Check sheet for the drawn part. Datum: minimum x, y, z corner. Units: mm. A direction names the side the tool comes from. Give positions to 0.01 mm unless a question says otherwise; leave off trailing zeros.
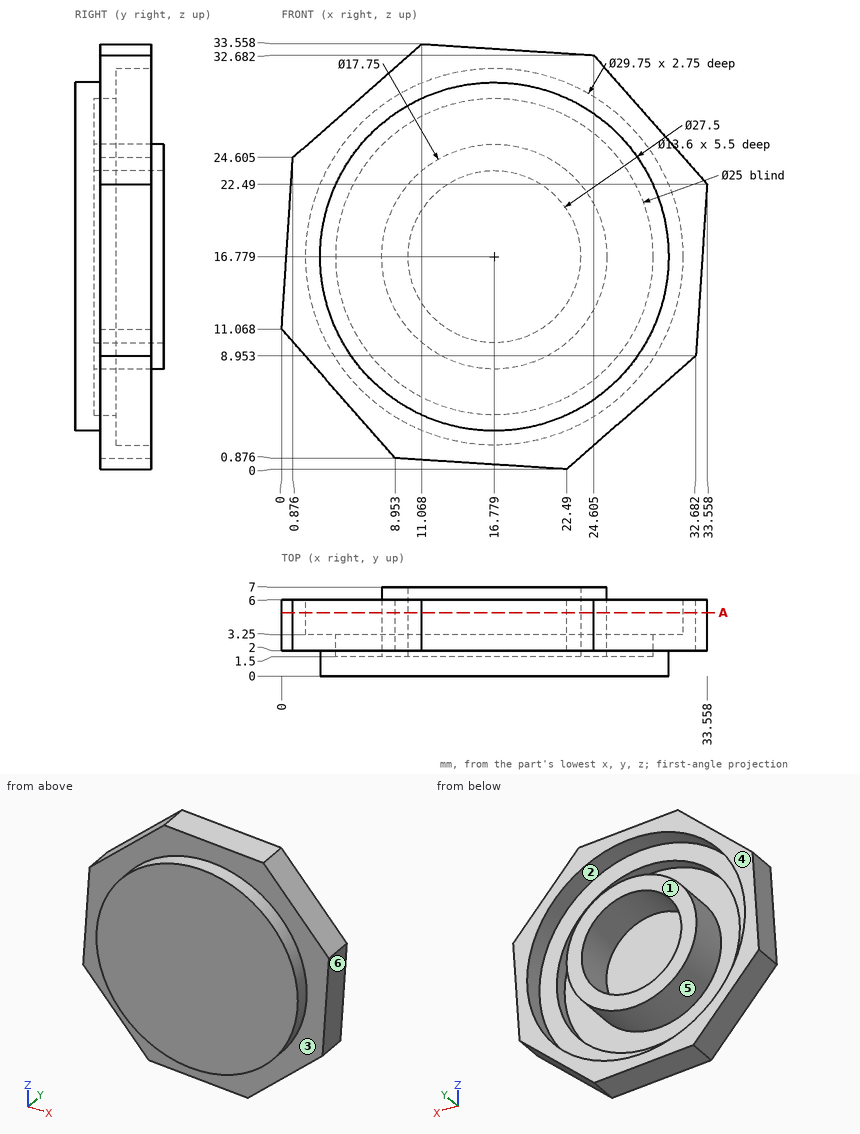
(1) Section check A-A, the plane y = 5. Give the number of separate pieces and of enclosed holes in the cut face.
Solved:
separate pieces: 2
enclosed holes: 2
(2) Scan lines: line 1 (X direction, y = 4.5, z = 14.5) (1 decimal); line 2 (X direction, y = 3.5, z = 15) (1 decimal); line 3 (Z direction, x = 16, y = 5.5) (1 decimal). Record each from-to range of solid material in increasing order.
Solved:
line 1: x = 0.2 to 2.1, 8.2 to 10.4, 23.2 to 25.4, 31.5 to 33
line 2: x = 0.3 to 2, 8.1 to 10.2, 23.3 to 25.5, 31.5 to 33.1
line 3: z = 0.4 to 1.9, 7.9 to 10, 23.5 to 25.6, 31.6 to 33.2
(3) Go/stop test with flat-tipped pins: pin 1 (4 mm diameter, centred on x = 15, y = 2, fed in from -Z) (1 decimal); pin 2 (1 mm diameter, centred on x = 24, y = 4, fed in from -Z); pin 3 (2 mm diameter, centred on y = 2.5, z = 27.5, fed in from -X) (1 decimal). Record where each tip stops, or that it passes through.
Solved:
pin 1: stops at z = 0.4
pin 2: stops at z = 0.89
pin 3: stops at x = 3
(4) Set-up check for the marked faces 1, 2 and 3: record each of +Z, -Z, +X, -X, +Y, -Y from which the full face is reachable in a straight line by a thin tool's end or side.
Solved:
face 1: +Z, -Z, +X, -X, +Y
face 2: +Y
face 3: -Y
(5) Release check for a two-part mould opening along Z. For the marked faces 4, 5 and 6 record: pulls with the +Z half, pulls with the -Z half, needs draft (parallel to the pull), parting line crosses it, or undercut.
Solved:
face 4: needs draft
face 5: undercut
face 6: pulls with the -Z half
